Geometry: final body of the model. Coordinates: model frame, mm. A direction names the side the tool comes from. Round coordinates to 2 decimals unless told otherwise and drop trailing zeros. Loops run counter-clockwise (first coordinate to the right, second up) from the corner with the lowest first, then second, coordinate; pieces in that order, holes last. Notation, with made-up numbers: M 24,-16.75 L 41,-16.75 A22 cw 41,11.25 Z; hole C -4.75,54.5 d11. An arc over 180 degrees is marked long. Return JSON: item names as keys, results as strings.
from build123d import *

# Parameters (mm, degrees)
F1_DEPTH  = 31.75
F3_DEPTH  = 25.4
F5_DEPTH  = 31.75
F7_R      = 31.75
F8_R      = 9.525
F9_R      = 3.175
F10_R     = 6.35
F11_DEPTH = 6.35


with BuildPart() as f1:
    # F0 (on Top) → F1 (new body)
    with BuildSketch(Plane.XY):
        with BuildLine():
            Line((123.825, 15.875), (0, 15.875))
            ThreePointArc((0, 15.875), (-15.875, 0), (0, -15.875))
            Line((0, -15.875), (104.775, -15.875))
            Line((104.775, -15.875), (104.775, -9.525))
            Line((104.775, -9.525), (0, -9.525))
            ThreePointArc((0, -9.525), (-9.525, 0), (0, 9.525))
            Line((0, 9.525), (123.825, 9.525))
            Line((123.825, 9.525), (123.825, 15.875))
        make_face()
    extrude(amount=F1_DEPTH)

    # F2 (on face) → F3 (cut)
    with BuildSketch(Plane.XZ.offset(-9.525)):
        Polygon((123.825, 31.75), (90.829432, 31.75), (123.825, 12.7), align=None)
    extrude(amount=-F3_DEPTH, mode=Mode.SUBTRACT)


with BuildPart() as f5:
    # F4 (on face) → F5 (new body)
    with BuildSketch(Plane.YZ.offset(104.775)):
        Polygon((-15.875, 57.15), (-15.875, 50.8), (-15.875, 31.75), (-9.525, 31.75), (-9.525, 50.8), (15.875, 50.8), (15.875, 57.15), align=None)
    extrude(amount=-F5_DEPTH)


with BuildPart() as f1_1:
    add(f1.part)

    # F6: union F5
    add(f5.part)

    # F7
    f7_edges = [f1_1.edges().sort_by_distance(p)[0] for p in [
        (104.775, -12.7, 0),
    ]]
    fillet(f7_edges, radius=F7_R)

    # F8
    f8_edges = [f1_1.edges().sort_by_distance(p)[0] for p in [
        (88.9, -15.875, 57.15),
    ]]
    fillet(f8_edges, radius=F8_R)

    # F9
    f9_edges = [f1_1.edges().sort_by_distance(p)[0] for p in [
        (88.9, -9.525, 50.8),
    ]]
    fillet(f9_edges, radius=F9_R)

    # F10 (on face) → F11 (cut)
    with BuildSketch(Plane.XZ.offset(15.875)):
        with Locations((12.7, 15.875)):
            Circle(F10_R)
        with Locations((47.625, 15.875)):
            Circle(F10_R)
    extrude(amount=-F11_DEPTH, mode=Mode.SUBTRACT)


solid = f1_1.part
Q1. Section query D-D (z = 28). Output: boundary loops of the cut face in (x, y) (3 decimals), plus the area to 3 significant figures.
Determined:
{"outline": "M 0,-15.875 L 104.553,-15.875 L 104.553,-9.525 L 0,-9.525 A9.525 cw 0,9.525 L 97.325,9.525 L 97.325,15.875 L 0,15.875 A15.875 ccw Z", "area": "1,540 mm^2"}
Q2. Section query A-A (y = 0). Output: boundary loops of the cut face in (x, z) (3 decimals), plus the area to 3 significant figures.
Determined:
{"outline": "M -15.875,0 L -9.525,0 L -9.525,31.75 L -15.875,31.75 Z; M 73.025,50.8 L 104.775,50.8 L 104.775,57.15 L 73.025,57.15 Z", "area": "403 mm^2"}
Q3. Material intervals for L1, parallel to Z at x = 12.7, y = -14 (3 decimals); L2, parallel to Y at x = 98, z = 23.5 (3 decimals); L3, parallel to Z at x = 91.5, y = 1, sorted ascending.
Determined:
{"L1": "z = 0 to 9.525, 22.225 to 31.75", "L2": "y = -15.875 to -9.525, 9.525 to 15.875", "L3": "z = 50.8 to 57.15"}
Q4. Section query C-C (x = 67.5). Output: boundary loops of the cut face in (y, z) (3 decimals), plus the area to 3 significant figures.
Determined:
{"outline": "M -15.875,0 L -9.525,0 L -9.525,31.75 L -15.875,31.75 Z; M 9.525,0 L 15.875,0 L 15.875,31.75 L 9.525,31.75 Z", "area": "403 mm^2"}
Q5. Pull-direction query (Y, two-part tool) for faces 5 (the flat face through (61, 9.525, 16)), 6 (the flat face through (37, 11, 0)), 7 (the cylindrical face through (88.678, -8.62, 49.845)), 8 (the flat face through (53, -9.525, 23)); classes: pulls with the +Y half, pulls with the -Y half, needs draft (parallel to the pull), parting line crosses it, or undercut.
Determined:
{"face 5": "undercut", "face 6": "needs draft", "face 7": "pulls with the +Y half", "face 8": "undercut"}
Q6. Section query B-B (x = 12.7). Output: boundary loops of the cut face in (y, z) (3 decimals).
Determined:
{"outline": "M -15.875,0 L -9.525,0 L -9.525,9.525 L -15.875,9.525 Z; M -15.875,22.225 L -9.525,22.225 L -9.525,31.75 L -15.875,31.75 Z; M 9.525,0 L 15.875,0 L 15.875,31.75 L 9.525,31.75 Z"}
Q7. Pin query (flat end, axial travel): pin 1 (3 mm diameter, centred on y = -2, z = 6, fed in from -X); pin 2 (6 mm diameter, centred on x = 105.5, y = -12.5, fed in from +Z). Return the tip coordinate at first contact, or that it passes through.
Determined:
{"pin 1": "stops at x = -15.87", "pin 2": "stops at z = 56.58"}
Q8. Reachability of faces 1 (the flat face through (107.096, 12.656, 22.358)), 2 (the cylindrical face through (95.721, -12.656, 9.548)), 3 (the flat face through (89, 5, 50.8)), 4 (the cylindrical face through (7.66, -12.74, 12.01)) from +Z, -Z, +X, -X, +Y, -Y: full face, straight path, thin tool, end or side. Return the list, or none.
Determined:
{"face 1": "+X, +Y", "face 2": "-Z, +X, -Y", "face 3": "+X, -X, +Y", "face 4": "-Y"}
